The model under review builds one solid part; all positions refer to its coordinate system, in mm. Face numbers are marked on the shaded views. Coordinates: 2 decimals unless noted, no trailing zeros. Order: outer loops, then holes, each group sorted by start corner. A loop starts at its lowest first (then second) coordinate and runs counter-clockwise, first axis right, second up. Notation, with made-up numbers: (27, 1) -> (71, 1) arc R26 cw to (71, 22) -> close; hole circle Ø5 at (-0.5, 10). An arc over 180 degrees is marked (long way). Use one line per item in the form item = value. Start each with the question number.
(1) Insertion check: pin 1 Ø6 at (x, z) = (19.5, 14.5) entering from -Y; pin 2 Ø8 at (y, z) = (6, -3) entering from +X; pin 3 Ø1.1 at (y, z) = (13, -6.5) entering from -X. Each pin has a flat end and moves straight along its axis. Give the tip position at first contact, or say it passes through.
(2) Take a section at D-D (x = 47). State the section outline as (y, z) points.
(3) Wall thickness on line 1 along Z through (x, y) = (20, 8); line 2 along Z through (x, y) = (24, 5); line 3 along Z through (x, y) = (47, 9.5): over which ranges is each line inside the solid? List them lowest first.
(4) Mouldability with a two-part tool opening along Y and no side actions: class the marked faces 1, 2, 3 and 4 as +Y half, -Y half, draft (parallel to the pull), parting line (faces both ways), or undercut.
(5) Take a section at C-C (z = 20). State the section outline as (x, y) points.
(6) Take a section at A-A (x = 34). State the section outline as (y, z) points, then the cut area to 3 significant figures.
(7) Take a section at B-B (y = 8). State the section outline as (x, z) points (3 decimals), then the cut area to 3 significant figures.
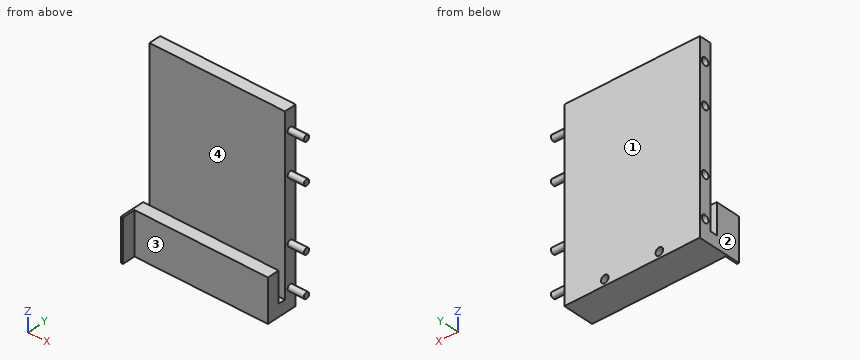
```python
from build123d import *

# Parameters (mm, degrees)
F1_DEPTH  = 67
F2_R      = 1.5
F3_DEPTH  = 8
F4_R      = 1.875
F5_DEPTH  = 9
F6_R      = 1.875
F7_DEPTH  = 9
F8_W      = 1
F8_H      = 21
F9_DEPTH  = 6.5
F10_R     = 1.875
F11_DEPTH = 9


# Not quite as in the source:
# - a feature names something its author has since deleted; it is built from what else it names


with BuildPart() as f1:
    # F0 (on Right) → F1 (new body)
    with BuildSketch(Plane.YZ):
        Polygon((14.9777059274, -37.1211464703), (14.9777059274, 53.8788535297), (8.9777059274, 53.8788535297), (8.9777059274, -31.1211464703), (5.4777059274, -31.1211464703), (5.4777059274, -16.1211464703), (-0.5222940726, -16.1211464703), (-0.5222940726, -37.1211464703), align=None)
    extrude(amount=F1_DEPTH)

    # F2 (on face) → F3 (join)
    with BuildSketch(Plane.YZ.offset(67)):
        with BuildLine():
            Line((11.9777059274, 43.8788535297), (11.9777059274, 45.3788535297))
            ThreePointArc((11.9777059274, 45.3788535297), (10.4777059274, 43.8788535297), (11.9777059274, 42.3788535297))
            Line((11.9777059274, 42.3788535297), (11.9777059274, 43.8788535297))
        make_face()
        with BuildLine():
            ThreePointArc((11.9777059274, 42.3788535297), (13.0383660992, 42.8181933579), (13.4777059274, 43.8788535297))
            ThreePointArc((13.4777059274, 43.8788535297), (13.0383660992, 44.9395137015), (11.9777059274, 45.3788535297))
            Line((11.9777059274, 45.3788535297), (11.9777059274, 43.8788535297))
            Line((11.9777059274, 43.8788535297), (11.9777059274, 42.3788535297))
        make_face()
        with BuildLine():
            ThreePointArc((13.4777059274, 23.8788535297), (13.0383660992, 24.9395137015), (11.9777059274, 25.3788535297))
            ThreePointArc((11.9777059274, 25.3788535297), (10.9170457557, 22.8181933579), (13.4777059274, 23.8788535297))
        make_face()
        with Locations((11.9777059274, -7.1211464703)):
            Circle(F2_R)
        with Locations((11.9777059274, -27.1211464703)):
            Circle(F2_R)
    extrude(amount=F3_DEPTH)

    # F4 (on face) → F5 (cut)
    with BuildSketch(Plane(origin=(0, 0, 0), x_dir=(0, -1, 0), z_dir=(-1, 0, 0))):
        with Locations((-18.4777059274, 23.8788535297)):
            Circle(F4_R)
        with Locations((-18.4777059274, 43.8788535297)):
            Circle(F4_R)
        with Locations((-18.4777059274, -7.1211464703)):
            Circle(F4_R)
        with Locations((-18.4777059274, -27.1211464703)):
            Circle(F4_R)
    extrude(amount=-F5_DEPTH, mode=Mode.SUBTRACT)

    # F6 (on face) → F7 (cut)
    with BuildSketch(Plane(origin=(0, 14.9777059274, 0), x_dir=(-1, 0, 0), z_dir=(0, 1, 0))):
        with Locations((-47, -34.1211464703)):
            Circle(F6_R)
        with Locations((-20, -34.1211464703)):
            Circle(F6_R)
    extrude(amount=-F7_DEPTH, mode=Mode.SUBTRACT)

    # F8 (on face) → F9 (join)
    with BuildSketch(Plane.XZ.offset(0.5222940726)):
        with Locations((0.5, -26.6211464703)):
            Rectangle(F8_W, F8_H)
    extrude(amount=F9_DEPTH)

    # F10 (on face) → F11 (cut)
    with BuildSketch(Plane(origin=(0, 0, 0), x_dir=(0, -1, 0), z_dir=(-1, 0, 0))):
        with BuildLine():
            ThreePointArc((-10.1027059274, 43.8788535297), (-10.6518807127, 45.2046787444), (-11.9777059274, 45.7538535297))
            Line((-11.9777059274, 45.7538535297), (-11.9777059274, 43.8788535297))
            Line((-11.9777059274, 43.8788535297), (-11.9777059274, 42.0038535297))
            ThreePointArc((-11.9777059274, 42.0038535297), (-10.6518807127, 42.553028315), (-10.1027059274, 43.8788535297))
        make_face()
        with BuildLine():
            ThreePointArc((-10.1027059274, 23.8788535297), (-10.6518807127, 25.2046787444), (-11.9777059274, 25.7538535297))
            ThreePointArc((-11.9777059274, 25.7538535297), (-13.3035311422, 22.553028315), (-10.1027059274, 23.8788535297))
        make_face()
        with BuildLine():
            Line((-11.9777059274, 43.8788535297), (-11.9777059274, 45.7538535297))
            ThreePointArc((-11.9777059274, 45.7538535297), (-13.8527059274, 43.8788535297), (-11.9777059274, 42.0038535297))
            Line((-11.9777059274, 42.0038535297), (-11.9777059274, 43.8788535297))
        make_face()
        with Locations((-11.9777059274, -27.1211464703)):
            Circle(F10_R)
        with Locations((-11.9777059274, -7.1211464703)):
            Circle(F10_R)
    extrude(amount=-F11_DEPTH, mode=Mode.SUBTRACT)


solid = f1.part
```
Findings:
q1.pin_1 = 8.98
q1.pin_2 = 67
q1.pin_3 = 9
q2.outline = (-0.52, -37.12) -> (14.98, -37.12) -> (14.98, -36) -> (5.98, -36) -> (5.98, -32.25) -> (14.98, -32.25) -> (14.98, 53.88) -> (8.98, 53.88) -> (8.98, -31.12) -> (5.48, -31.12) -> (5.48, -16.12) -> (-0.52, -16.12) -> close
q3.line_1 = -37.12 to -36, -32.25 to -31.12
q3.line_2 = -37.12 to -16.12
q3.line_3 = -37.12 to -36, -32.25 to 53.88
q4.face_1 = +Y half
q4.face_2 = draft
q4.face_3 = -Y half
q4.face_4 = undercut
q5.outline = (0, 8.98) -> (67, 8.98) -> (67, 14.98) -> (0, 14.98) -> close
q6.outline = (-0.52, -37.12) -> (14.98, -37.12) -> (14.98, 53.88) -> (8.98, 53.88) -> (8.98, -31.12) -> (5.48, -31.12) -> (5.48, -16.12) -> (-0.52, -16.12) -> close
q6.area = 693 mm²
q7.outline = (0, -37.121) -> (67, -37.121) -> (67, -31.121) -> (0, -31.121) -> close; hole circle Ø3.75 at (20, -34.121); hole circle Ø3.75 at (47, -34.121)
q7.area = 380 mm²
